Autodesk Inventor part; units mm, degrees
ref_plane "YZ Plane" through (0, 0, 0) normal (1, 0, 0) x (0, 1, 0)
ref_plane "XZ Plane" through (0, 0, 0) normal (0, 1, 0) x (-1, 0, 0)
ref_plane "XY Plane" through (0, 0, 0) normal (0, 0, 1) x (1, 0, 0)
sketch "Skizze1" plane through (0, 0, 0) normal (0, 1, 0) x (-1, 0, 0)
  line L0 (-5, -25) -> (5, -25)
  line L1 (5, -25) -> (5, 25)
  line L2 (5, 25) -> (-5, 25)
  line L3 (-5, 25) -> (-5, -25)
  line L4 (-5, -25) -> (5, 25) construction
  line L5 (5, -25) -> (-5, 25) construction
  point P0 (0, 0)
  dimension "d0" = 10
  dimension "d1" = 50
extrude "Extrusion1" add sketch "Skizze1" along normal blind 10
sketch "Skizze2" plane through (-5, 0, 25) normal (0, 0, 1) x (1, 0, 0)
  circle A0 centre (5, 5) radius 0.8
  point P0 (5, 0)
  dimension "d4" = 1.6
hole "Bohrung1" at (0, 5, 25) direction (0, 0, -1) diameter 1.6 end through all
sketch "Skizze3" plane through (0, 10, 0) normal (0, 1, 0) x (1, 0, 0)
  point P0 (0, 0)
sketch "Skizze4" plane through (0, 10, 0) normal (0, 1, 0) x (1, 0, 0)
  point P0 (0, 0)
sketch "Skizze5" plane through (0, 10, 0) normal (0, 1, 0) x (1, 0, 0)
  line L0 (-5, 25) -> (-5, -25)
  line L1 (5, -25) -> (5, 25)
  line L2 (-5, -25) -> (5, -25)
  line L3 (5, -25) -> (5, 25)
  line L4 (5, 25) -> (-5, 25)
  line L5 (-5, 25) -> (-5, -25)
  point P0 (0, 0)
extrude "Extrusion2" add sketch "Skizze5" along normal blind 2
sketch "Skizze6" plane through (0, 12, 0) normal (0, 1, 0) x (1, 0, 0)
  point P0 (0, 0)
hole "Bohrung2" at (0, 12, 0) direction (0, -1, 0) diameter 1 depth 6.7
sketch "Skizze7" plane through (0, 12, 0) normal (0, 1, 0) x (1, 0, 0)
  point P0 (0, 0)
hole "Bohrung3" at (0, 12, 0) direction (0, -1, 0) diameter 5.4 depth 5.7
sketch "Skizze8" plane through (-5, 0, 25) normal (0, 0, 1) x (1, 0, 0)
  circle A0 centre (5, 5.0108) radius 1.4918
  point P0 (5, 0)
hole "Bohrung4" at (0, 5.0108, 25) direction (0, 0, -1) diameter 5.4 depth 5.7
sketch "Skizze9" plane through (5, 0, -25) normal (0, 0, -1) x (-1, 0, 0)
  circle A0 centre (5, 5) radius 0.8
  circle A1 centre (5, 5) radius 2.7
  point P0 (5, 0)
  dimension "d35" = 5.4
hole "Bohrung5" at (0, 5, -25) direction (0, 0, 1) diameter 5.4 depth 5.7
properties part number "T-Sensor_PT100" material "PMMA-Kunststoff"
Could you check a few things on this model? Use its own coordinates, in mm. A direction names the side the tool comes from. Round coordinates to 2 decimals unless told otherwise and drop trailing zeros. Loops run counter-clockwise (first coordinate to the right, second up) from the corner with the lowest first, then second, coordinate; pieces in that order, holes last. Notation, with made-up numbers: M -18.75,-7.75 L 4.25,-7.75 A14 ccw 4.25,17.25 Z; hole C 40,4.5 d3. An arc over 180 degrees is marked long. Put each result on its own line as item: value.
Q1. For pin 1 (4.5 mm diameter, centred on x = 0, z = -1, fed in from +Y); pin 2 (2.5 mm diameter, centred on x = -1, y = 5, fed in from +Z), each with a flat end and sliding along its axis, tell me the tip position at first contact or that it passes through.
Check result:
pin 1: y = 12
pin 2: z = 19.3
Q2. Imagine slicing it at A-A (y = 5). Write out the boundary of the cut face in (x, z), then the cut area to 3 significant figures.
Check result:
outline: M -5,-25 L -2.7,-25 L -2.7,-19.3 L -0.8,-19.3 L -0.8,19.3 L -2.7,19.3 L -2.7,25 L -5,25 Z; M 0.8,-19.3 L 2.7,-19.3 L 2.7,-25 L 5,-25 L 5,25 L 2.7,25 L 2.7,19.3 L 0.8,19.3 Z
area: 377 mm2
Q3. Imagine slicing it at D-D (x = -1.25). Write out the boundary of the cut face in (y, z), then the cut area to 3 significant figures.
Check result:
outline: M 0,-25 L 2.61,-25 L 2.61,-19.3 L 7.39,-19.3 L 7.39,-25 L 12,-25 L 12,-2.39 L 6.3,-2.39 L 6.3,2.39 L 12,2.39 L 12,25 L 7.4,25 L 7.4,19.3 L 2.62,19.3 L 2.62,25 L 0,25 Z
area: 518 mm2
Q4. Thinking about a two-plate mould opening in Z: for faces 1 (the face through (-0.3, 6, -0.4)), 2 (the face through (0, 9, 25)), 3 (the face through (0, 9, -25)), which applies, released by +Z, released by -Z, zero draft, split by the parting line, or undercut?
Check result:
face 1: undercut
face 2: released by +Z
face 3: released by -Z
Q5. Imagine slicing it at C-C (z = 18.5). Write out the boundary of the cut face in (x, y).
Check result:
outline: M -5,0 L 5,0 L 5,12 L -5,12 Z; hole C 0,5 d1.6
Q6. Imagine slicing it at B-B (z = 0). Write out the boundary of the cut face in (x, y).
Check result:
outline: M -5,0 L 5,0 L 5,12 L 2.7,12 L 2.7,6.3 L 0.5,6.3 L 0.5,5.62 A0.8 cw long -0.5,5.62 L -0.5,6.3 L -2.7,6.3 L -2.7,12 L -5,12 Z
Q7. I need wall thicknesses on probe 1 along X at (y, z) = (5, -6.5); probe 2 along X at (y, z) = (6, 0); probe 3 along Z at (x, y) = (0, 9.6). Which ranges of each line are inside material? Lowest first, please.
Check result:
probe 1: -5 to -0.8, 0.8 to 5
probe 2: -5 to -0.5, 0.5 to 5
probe 3: -25 to -2.7, 2.7 to 25
Q8. On a 3-axis mill with a long thin cutter (end or side, diameter ignored), from which of +Z, -Z, +X, -X, +Y, -Y can I reach the whole of each face in a straight line? I mean faces 4 (the face through (1, 6.3, 0)), 5 (the face through (-0.24, 4.237, -0.27)), 6 (the face through (1, 4, -19.3)), 7 (the face through (-1, 4, 19.3)). Say none if no direction works.
Check result:
face 4: +Y
face 5: +Z, -Z
face 6: -Z
face 7: +Z
